Can you work these out from the model? Positions are in its coordinate system, mm. Face numbers are marked on the shaded views. A direction names the side the tool comes from. Give positions to 0.01 mm unless a question says otherwise; leave off trailing zeros. Loops run counter-clockwise (first coordinate to the right, second up) from the corner with the lowest first, then second, coordinate; pieces in that order, holes last. Notation, with made-up numbers: (32, -11) -> (62, -11) arc R23 cw to (62, 11) -> close; hole circle Ø5 at (23, 67). An arc over 180 degrees is marked (long way). Return JSON: item names as keys, results as strings. Group by question number.
Q1. Suppose I cut it at D-D, the plane z = -0.75. Please give me the cut outline in (x, y), and give its area (3 significant figures).
Q2. I need wall thicknesses on line 1 along X through (y, z) = (0, -8.15); line 2 along Y through (x, z) = (0, -7.35); line 3 along Z through (x, y) = (1.5, -2.75). Which ranges of each line are inside material? Lowest first, please. Write a range as [from, to].
Q3. Thinking about a two-plate mould opening in Y: for the marked faces 5, 6, 7 and 8, which applies, pulls with the +Y half, pulls with the -Y half, needs draft (parallel to the pull), parting line crosses it, or undercut?
Q4. Suppose I cut it at C-C, the plane z = -5.25. Please give me the cut outline in (x, y).
Q5. Will these pins go through, and if not, where does the flat tip stop? pin 1 (6 mm diameter, centred on x = -6.5, z = -5, fed in from +Y); pin 2 (2 mm diameter, centred on x = 4.5, z = -6.5, fed in from +Y); pin 3 (6 mm diameter, centred on x = -4.5, y = -6.5, fed in from +Z).
Q6. Suppose I cut it at A-A, the plane x = 0. Please give me the cut outline in (y, z), and give its area (3 significant figures).
Q7. Which directions (+Z, -Z, +X, -X, +Y, -Y) give clear straight access to the entire face, cutting with the end or side of a thin tool? Please do the marked faces 1, 2, 3 and 4.
Q8. Suppose I cut it at B-B, the plane y = -6.75. Please give me the cut outline in (x, z).
```python
from build123d import *

# Parameters (mm, degrees)
CUT_EXTRUDE1_DEPTH      = 6
CUT_EXTRUDE1_DEPTH_BACK = 6


with BuildPart() as part:
    # Sketch1 → Revolve1 (revolve)
    with BuildSketch(Plane(origin=(0, 0, 0), x_dir=(0, 0, -1), z_dir=(1, 0, 0))):
        with BuildLine():
            Line((0, 1.75), (0, 3.25))
            Line((0, 3.25), (1, 3.25))
            ThreePointArc((1, 3.25), (3.121320344, 4.128679656), (4, 6.25))
            Line((4, 6.25), (4, 10))
            Line((4, 10), (5, 10))
            Line((5, 10), (5, 8.5))
            Line((5, 8.5), (10, 8.5))
            Line((10, 8.5), (10, 7))
            Line((10, 7), (5, 7))
            Line((5, 7), (5, 1.75))
            Line((5, 1.75), (0, 1.75))
        make_face()
    revolve(axis=Axis((0, 0, 0), (0, 0, -1)))

    # Sketch2 → Cut-Extrude1 (cut, two sides)
    with BuildSketch(Plane(origin=(0, 0, -5), x_dir=(-1, 0, 0), z_dir=(0, 0, -1))) as cut_extrude1_sk:
        with BuildLine():
            Line((-1.75, 9.845684334), (-1.75, 6.777720856))
            ThreePointArc((-1.75, 6.777720856), (0, 7), (1.75, 6.777720856))
            Line((1.75, 6.777720856), (1.75, 9.845684334))
            ThreePointArc((1.75, 9.845684334), (0, 10), (-1.75, 9.845684334))
        make_face()
        with BuildLine():
            Line((-1.75, 6.777720856), (-1.75, 0))
            ThreePointArc((-1.75, 0), (0, 1.75), (1.75, 0))
            Line((1.75, 0), (1.75, 6.777720856))
            ThreePointArc((1.75, 6.777720856), (0, 7), (-1.75, 6.777720856))
        make_face()
    extrude(amount=CUT_EXTRUDE1_DEPTH, mode=Mode.SUBTRACT)
    extrude(cut_extrude1_sk.sketch, amount=-CUT_EXTRUDE1_DEPTH_BACK, mode=Mode.SUBTRACT)


solid = part.part
```
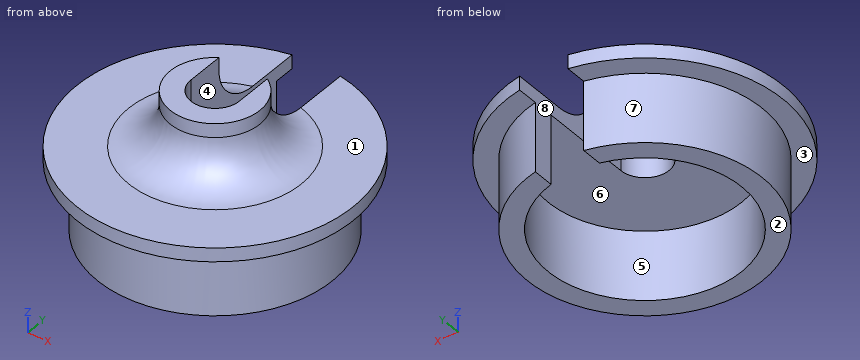
Ans:
{
 "1": {"outline": "(-1.75, 0) -> (-1.75, 2.74) arc R3.25 ccw (long way) to (1.75, 2.74) -> (1.75, 0) arc R1.75 cw to start", "area": "17.6 mm^2"},
 "2": {"line 1": "x = [-8.5, -7], [7, 8.5]", "line 2": "y = [-8.5, -7]", "line 3": "z = [-5, 0]"},
 "3": {"face 5": "undercut", "face 6": "undercut", "face 7": "parting line crosses it", "face 8": "needs draft"},
 "4": {"outline": "(-1.75, 6.78) -> (-1.75, 8.32) arc R8.5 ccw (long way) to (1.75, 8.32) -> (1.75, 6.78) arc R7 cw (long way) to start"},
 "5": {"pin 1": "stops at y = 9.37", "pin 2": "stops at y = 7.75", "pin 3": "stops at z = -3.68"},
 "6": {"outline": "(-10, -5) -> (-8.5, -5) -> (-8.5, -10) -> (-7, -10) -> (-7, -5) -> (-1.75, -5) -> (-1.75, 0) -> (-3.25, 0) -> (-3.25, -1) arc R3 cw to (-6.25, -4) -> (-10, -4) -> close", "area": "23.7 mm^2"},
 "7": {"face 1": "+Z", "face 2": "-Z, +X, -X, +Y, -Y", "face 3": "-Z", "face 4": "+Z, -Z, +Y"},
 "8": {"outline": "(-7.38, -5) -> (-5.17, -5) -> (-5.17, -10) -> (-1.85, -10) -> (-1.85, -5) -> (1.85, -5) -> (1.85, -10) -> (5.17, -10) -> (5.17, -5) -> (7.38, -5) -> (7.38, -4) -> (-7.38, -4) -> close"}
}
